```python
from build123d import *

# Parameters (mm, degrees)
FILLET_1_R          = 2
SKETCH_2_R          = 7.321356554
SKETCH_2_W          = 2
SKETCH_2_H          = 11.961651185
CUT_EXTRUDE_1_DEPTH = 11
CUT_EXTRUDE_2_REACH = 53.945
SKETCH_3_R          = 1.5
FILLET_2_R          = 0.2
FILLET_3_R          = 0.5
FILLET_4_R          = 0.5


with BuildPart() as part:
    # 草图1 → 旋转1 (revolve)
    with BuildSketch(Plane.XY):
        Polygon((0, 0), (0, 3), (-29, 3), (-29, 5), (-39, 5), (-39, 4.5), (-51, 4.5), (-51, 0), align=None)
    revolve(axis=Axis((0, 0, 0), (-1, 0, 0)))

    # 圆角1
    fillet_1_edges = [part.edges().sort_by_distance(p)[0] for p in [
        (-51, -4.5, 0),
    ]]
    fillet(fillet_1_edges, radius=FILLET_1_R)

    # 草图2 → 切除-拉伸1 (cut)
    with BuildSketch(Plane.ZY.offset(51)):
        Circle(SKETCH_2_R)
        with Locations((2.5, -0.178000761)):
            Rectangle(SKETCH_2_W, SKETCH_2_H, mode=Mode.SUBTRACT)
        with Locations((-2.5, -0.178000761)):
            Rectangle(SKETCH_2_W, SKETCH_2_H, mode=Mode.SUBTRACT)
    extrude(amount=-CUT_EXTRUDE_1_DEPTH, mode=Mode.SUBTRACT)

    # 切除-拉伸2: up to this face of the body (flat: up to its plane)
    cut_extrude_2_end = Plane(part.part.faces().sort_by_distance((-45.204174513, -1.4e-08, -3.5))[0])
    # 草图3 → 切除-拉伸2 (cut, up to the picked face)
    with BuildSketch(Plane.XY.offset(3.5), mode=Mode.PRIVATE) as cut_extrude_2_sk1:
        with Locations(Location((-46, 0, 0), (0, 0, 270))):
            Circle(SKETCH_3_R)
    cut_extrude_2_tool1 = split(extrude(cut_extrude_2_sk1.sketch, amount=-CUT_EXTRUDE_2_REACH, mode=Mode.PRIVATE), bisect_by=cut_extrude_2_end, keep=Keep.BOTH, mode=Mode.PRIVATE)
    add(cut_extrude_2_tool1.solids().sort_by(Axis((-46, 0, 3.5), (0, 0, -1)))[0], mode=Mode.SUBTRACT)

    # 圆角2
    fillet_2_edges = [part.edges().sort_by_distance(p)[0] for p in [
        (-39, -4.5, 0),
    ]]
    fillet(fillet_2_edges, radius=FILLET_2_R)

    # 圆角3
    fillet_3_edges = [part.edges().sort_by_distance(p)[0] for p in [
        (0, -3, 0),
    ]]
    fillet(fillet_3_edges, radius=FILLET_3_R)

    # 圆角4
    fillet_4_edges = [part.edges().sort_by_distance(p)[0] for p in [
        (-29, -5, 0),
        (-39, -5, 0),
    ]]
    fillet(fillet_4_edges, radius=FILLET_4_R)


solid = part.part
```
Check sheet for the modelled part. Datum: model origin and axes. Units: mm. A direction names the side the tool comes from. Give positions to 0.01 mm unless a question says otherwise; leave off trailing zeros. Order: outer loops, then holes, each group sorted by start corner. A loop starts at its lowest first (then second) coordinate and runs counter-clockwise, first axis right, second up. Notation, with made-up numbers: M -10,78.25 L -5,78.25 A24 ccw -5,112.25 Z; hole C 22.5,39 d11. An arc over 180 degrees is marked long. Answer in a Markdown table with one row per item. Add a question column.
Q1. Thickness scan on L1, parallel to X at y = 0, z = 2.4; L2, parallel to X at y = -1.25, z = 2.25; L3, parallel to Y at x = -35, z = 4. Record the ranges inside material, lowest first.
Q2. Sectioned sample at B-B, the plane y = 0. Count the separate pieces of the cut face and the enclosed holes in it, and give its area (3 significant figures).
Q3. Sectioned sample at A-A, the plane x = -42.5. Record the boundary of the cut face in (y, z).
Q4. Sectioned sample at C-C, the plane x = -31. Record the boundary of the cut face in (y, z).
Q5. Access from +Z, -Z, +X, -X, +Y, -Y to the whole of each face (thin tool, end or side, straight path). Record for faces 5 (the cylindrical face through (-43.1, -3.6, 2.7)), 6 (the flat face through (-29, -1, 3)), 7 (the flat face through (-44, 0, -3.5)).
Q6. Gauge pin test, flat ends, axial feed: pin 1 Ø4 at (x, y) = (-46.5, 0) entering from +Z; pin 2 Ø3 at (x, y) = (-13.5, 1) entering from +Z; pin 3 Ø1.7 at (x, y) = (-43.5, 0) entering from -Z. Record the tip position at first contact, or that the pin passes through.
Q7. Release check for a two-part mould opening along Z. For faces 1 (the flat face through (-40, 0, 0)), 2 (the cylindrical face through (-34.08, 4.77, -1.5)), 3 (the flat face through (-44, 0, -1.5)), 4 (the flat face through (-44, 0, 3.5)) record: released by +Z, released by -Z, zero draft, split by the parting line, or undercut.
Verdict:
| question | item | result |
|---|---|---|
| 1 | L1 | -51 to -47.5, -44.5 to 0 |
| 1 | L2 | -51 to -46.83, -45.17 to -0.01 |
| 1 | L3 | -3 to 3 |
| 2 | separate pieces | 3 |
| 2 | enclosed holes | 0 |
| 2 | area | 315 mm² |
| 3 | outline | M -4.24,-1.5 A4.5 ccw -2.83,-3.5 L 2.83,-3.5 A4.5 ccw 4.24,-1.5 Z; M -4.24,1.5 L 4.24,1.5 A4.5 ccw 2.83,3.5 L -2.83,3.5 A4.5 ccw Z |
| 4 | outline | C 0,0 d10 |
| 5 | face 5 | -X |
| 5 | face 6 | +X |
| 5 | face 7 | -Z, -X, +Y, -Y |
| 6 | pin 1 | z = 3.5 |
| 6 | pin 2 | z = 3 |
| 6 | pin 3 | z = -3.5 |
| 7 | face 1 | undercut |
| 7 | face 2 | split by the parting line |
| 7 | face 3 | undercut |
| 7 | face 4 | released by +Z |
